```python
from build123d import *

# Parameters (mm, degrees)
SKETCH1_W           = 20.2
SKETCH1_H           = 36.5
SKETCH1_W_2         = 12.2
SKETCH1_H_2         = 22.5
BOSS_EXTRUDE1_DEPTH = 22
SKETCH3_R           = 1
CUT_EXTRUDE2_DEPTH  = 0.0001
SKETCH6_W           = 14
SKETCH6_H           = 8
CUT_EXTRUDE3_DEPTH  = 25


with BuildPart() as part:
    # Sketch1 → Boss-Extrude1 (new body, symmetric)
    with BuildSketch(Plane(origin=(0, 0, 0), x_dir=(0, 0, -1), z_dir=(1, 0, 0))):
        Rectangle(SKETCH1_W, SKETCH1_H)
        Rectangle(SKETCH1_W_2, SKETCH1_H_2, mode=Mode.SUBTRACT)
    extrude(amount=BOSS_EXTRUDE1_DEPTH, both=True)

    # Sketch3 → Cut-Extrude2 (cut)
    with BuildSketch(Plane.XY.offset(10.1)):
        Circle(SKETCH3_R)
    extrude(amount=-CUT_EXTRUDE2_DEPTH, mode=Mode.SUBTRACT)

    # Sketch6 → Cut-Extrude3 (cut, symmetric)
    with BuildSketch(Plane(origin=(0, 0, 0), x_dir=(1, 0, 0), z_dir=(0, 1, 0))):
        Rectangle(SKETCH6_W, SKETCH6_H)
    extrude(amount=CUT_EXTRUDE3_DEPTH, both=True, mode=Mode.SUBTRACT)


solid = part.part
```
The model under review builds one solid part; all positions refer to its coordinate system, in mm. A direction names the side the tool comes from. Round coordinates to 2 decimals unless told otherwise and drop trailing zeros. Write each loop counter-clockwise with the first axis right and the second up, starting at its lowest first coordinate (ties: lowest second). Pieces come first, ordered by that corner, then holes.
(1) Mouldability with a two-part tool opening along Z and no side actions: class faces 4 (the flat face through (0, 4, 10.1)), 5 (the flat face through (0, 0, -10.1)), 6 (the flat face through (0, 15, 4)), 7 (the flat face through (22, 0, 7)) as +Z half, -Z half, draft (parallel to the pull), parting line (faces both ways), or undercut.
(2) We need section D-D on z = 4.5. Give the boundary of the cut face in (x, y).
(3) We need section A-A on y = -9.5. Give the boundary of the cut face in (x, z), and give its area (3 significant figures).
(4) Machinability: for faces 1 (the flat face through (0.3, 11.25, 4.2)), 2 (the flat face through (-7, -15, 0)), 3 (the flat face through (0, -18.25, 5)), which of the approach directions +Z, -Z, +X, -X, +Y, -Y give a long, thin tool a straight path to every point of the face, cutting with its end or side? Answer none if there is none.
(5) Wall thickness on L1, parallel to Z at x = -3.5, y = -5.5; L2, parallel to Y at x = 16.5, z = -1.5; L3, parallel to Z at x = -2.5, y = 16: over which ranges is each line inside the solid? List them lowest first.
(6) We need section B-B on z = 1.75. Give the boundary of the cut face in (x, y), and give its area (3 significant figures).
Findings below:
1. face 4: +Z half
1. face 5: -Z half
1. face 6: undercut
1. face 7: draft
2. outline: (-22, -18.25) - (22, -18.25) - (22, -11.25) - (-22, -11.25) - close; (-22, 11.25) - (22, 11.25) - (22, 18.25) - (-22, 18.25) - close
3. outline: (-22, -10.1) - (22, -10.1) - (22, -6.1) - (-22, -6.1) - close; (-22, 6.1) - (22, 6.1) - (22, 10.1) - (-22, 10.1) - close
3. area: 352 mm2
4. face 1: +X, -X
4. face 2: +Y, -Y
4. face 3: +Z, -Z, +X, -X, -Y
5. L1: z = -10.1 to -6.1, 6.1 to 10.1
5. L2: y = -18.25 to -11.25, 11.25 to 18.25
5. L3: z = -10.1 to -4, 4 to 10.1
6. outline: (-22, -18.25) - (-7, -18.25) - (-7, -11.25) - (-22, -11.25) - close; (-22, 11.25) - (-7, 11.25) - (-7, 18.25) - (-22, 18.25) - close; (7, -18.25) - (22, -18.25) - (22, -11.25) - (7, -11.25) - close; (7, 11.25) - (22, 11.25) - (22, 18.25) - (7, 18.25) - close
6. area: 420 mm2
